Geometry: final body of the model. Coordinates: model frame, mm. Give positions to 0.01 mm unless a question says otherwise; leave off trailing zeros. Write each loop counter-clockwise with the first axis right and the second up, starting at its lowest first coordinate (ties: lowest second). Pieces come first, ordered by that corner, then holes. Notation, with made-up numbers: M 48,74 L 105,74 A26 cw 105,96 Z; hole C 19.25,-18 d5. An arc over 180 degrees is marked long. Answer as a JSON object with one key per item and string values.
from build123d import *

# Parameters (mm, degrees)
SKETCH2_W           = 23
SKETCH2_H           = 35
SKETCH2_W_2         = 13
SKETCH2_H_2         = 23
BOSS_EXTRUDE1_DEPTH = 3.7
SKETCH3_R           = 0.8
CUT_EXTRUDE1_DEPTH  = 4.7
SKETCH5_W           = 10
SKETCH5_H           = 3.7
BOSS_EXTRUDE3_DEPTH = 19
SKETCH7_R           = 0.8
CUT_EXTRUDE2_DEPTH  = 4.7
FILLET1_R           = 5
FILLET2_R           = 2


with BuildPart() as part:
    # Sketch2 → Boss-Extrude1 (new body)
    with BuildSketch(Plane(origin=(0, 0, 0), x_dir=(1, 0, 0), z_dir=(0, 1, 0))):
        Rectangle(SKETCH2_W, SKETCH2_H)
        Rectangle(SKETCH2_W_2, SKETCH2_H_2, mode=Mode.SUBTRACT)
    extrude(amount=-BOSS_EXTRUDE1_DEPTH)

    # Sketch3 → Cut-Extrude1 (cut, through all)
    with BuildSketch(Plane(origin=(0, 0, 0), x_dir=(1, 0, 0), z_dir=(0, 1, 0))):
        with Locations((0, 14.5)):
            Circle(SKETCH3_R)
        with Locations((0, -14.5)):
            Circle(SKETCH3_R)
    extrude(amount=-CUT_EXTRUDE1_DEPTH, mode=Mode.SUBTRACT)

    # Sketch5 → Boss-Extrude3 (add)
    with BuildSketch(Plane(origin=(0, 0, -17.5), x_dir=(-1, 0, 0), z_dir=(0, 0, -1))):
        with Locations((0, -1.85)):
            Rectangle(SKETCH5_W, SKETCH5_H)
    extrude(amount=BOSS_EXTRUDE3_DEPTH)

    # Sketch7 → Cut-Extrude2 (cut, through all)
    with BuildSketch(Plane(origin=(0, 0, 0), x_dir=(1, 0, 0), z_dir=(0, 1, 0))):
        with Locations((0, 32.5)):
            Circle(SKETCH7_R)
        with Locations((0, 20.5)):
            Circle(SKETCH7_R)
    extrude(amount=-CUT_EXTRUDE2_DEPTH, mode=Mode.SUBTRACT)

    # Fillet1
    fillet1_edges = [part.edges().sort_by_distance(p)[0] for p in [
        (11.5, -1.85, 17.5),
        (-11.5, -1.85, 17.5),
        (-11.5, -1.85, -17.5),
        (11.5, -1.85, -17.5),
    ]]
    fillet(fillet1_edges, radius=FILLET1_R)

    # Fillet2
    fillet2_edges = [part.edges().sort_by_distance(p)[0] for p in [
        (5, -1.85, -17.5),
        (-5, -1.85, -17.5),
        (5, -1.85, -36.5),
        (-5, -1.85, -36.5),
    ]]
    fillet(fillet2_edges, radius=FILLET2_R)


solid = part.part
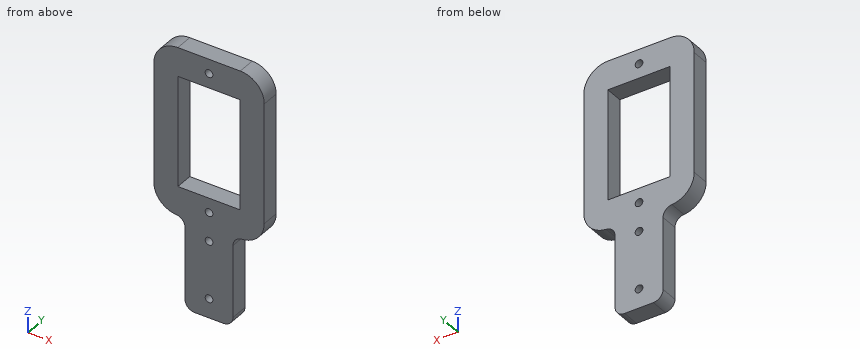
1) Cut plane A-A on x = -1.5. Return loops of the section in (y, z).
Geometry check:
{"outline": "M -3.7,-36.5 L 0,-36.5 L 0,-11.5 L -3.7,-11.5 Z; M -3.7,11.5 L 0,11.5 L 0,17.5 L -3.7,17.5 Z"}
2) Line query: line 1 (Z direction, x = 0, y = -1.9); line 2 (X direction, y = -1.3, z = -32.5); line 3 (X direction, y = -2.55, z = 4). Output: solid intervals per line, ascending. Write a range as from..to.
Geometry check:
{"line 1": "z = -36.5..-33.3, -31.7..-21.3, -19.7..-15.3, -13.7..-11.5, 11.5..13.7, 15.3..17.5", "line 2": "x = -5..-0.8, 0.8..5", "line 3": "x = -11.5..-6.5, 6.5..11.5"}
3) Cut plane D-D on z = -16. Return loops of the section in (x, y).
Geometry check:
{"outline": "M -10.07,-3.7 L 10.07,-3.7 L 10.07,0 L -10.07,0 Z"}
4) Cut plane B-B on z = 6.5. Return loops of the section in (x, y).
Geometry check:
{"outline": "M -11.5,-3.7 L -6.5,-3.7 L -6.5,0 L -11.5,0 Z; M 6.5,-3.7 L 11.5,-3.7 L 11.5,0 L 6.5,0 Z"}
5) Contact query for a flat-ended pin moving along its axis: P1, Ø1.9, axis at y = -1.5, z = -27.5, coming from the +X side. Output: stop coordinate, or through.
Geometry check:
{"P1": "stops at x = 5"}
6) Cut plane C-C on y = -2.8. Give the number of separate pieces and of enclosed holes in the cut face, and give its area (3 significant figures).
Geometry check:
{"separate pieces": "1", "enclosed holes": "5", "area": "666 mm2"}
